```python
from build123d import *

# Parameters (mm, degrees)
BOSS_EXTRUDE1_DEPTH    = 152.4
CONVERT_SOLID1_START   = -152.4
CONVERT_SOLID1_DEPTH   = 152.4
CONVERT_SOLID1_2_DEPTH = 152.4
SKETCH6_W              = 60.654765258
SKETCH6_H              = 35.589797731
CUT_EXTRUDE1_DEPTH     = 230.810351377
SKETCH7_W              = 82.570052287
SKETCH7_H              = 50.8
CUT_EXTRUDE2_DEPTH     = 180.914674499


# Read off the part's stored shape, not the designer's step: Convert-Solid1
with BuildPart() as part:
    # Sketch1 → Boss-Extrude1 (new body)
    with BuildSketch(Plane.XY):
        Polygon((-82.55, 0), (-82.55, 48.26), (82.55, 48.26), (82.55, 0), (81.28, 0), (81.28, 46.99), (-81.28, 46.99), (-81.28, 0), align=None)
    extrude(amount=-BOSS_EXTRUDE1_DEPTH)

    # Convert-Solid1 outline → Convert-Solid1 (cut)
    with BuildSketch(Plane.XY.offset(CONVERT_SOLID1_START)):
        with BuildLine():
            Line((82.55, 48.26), (80.01, 48.26))
            ThreePointArc((80.01, 48.26), (81.806051224, 47.516051224), (82.55, 45.72))
            Line((82.55, 45.72), (82.55, 48.26))
        make_face()
        with BuildLine():
            ThreePointArc((-82.55, 45.72), (-81.806051224, 47.516051224), (-80.01, 48.26))
            Line((-80.01, 48.26), (-82.55, 48.26))
            Line((-82.55, 48.26), (-82.55, 45.72))
        make_face()
    extrude(amount=CONVERT_SOLID1_DEPTH, mode=Mode.SUBTRACT)

    # Convert-Solid1 2 outline → Convert-Solid1 2 (add)
    with BuildSketch(Plane.XY.offset(CONVERT_SOLID1_START)):
        with BuildLine():
            Line((81.28, 46.99), (80.01, 46.99))
            ThreePointArc((80.01, 46.99), (80.908025612, 46.618025612), (81.28, 45.72))
            Line((81.28, 45.72), (81.28, 46.99))
        make_face()
        with BuildLine():
            ThreePointArc((-81.28, 45.72), (-80.908025612, 46.618025612), (-80.01, 46.99))
            Line((-80.01, 46.99), (-81.28, 46.99))
            Line((-81.28, 46.99), (-81.28, 45.72))
        make_face()
    extrude(amount=CONVERT_SOLID1_2_DEPTH)

    # Sketch6 → Cut-Extrude1 (cut, through all)
    with BuildSketch(Plane.ZY.offset(82.55)):
        with Locations((-1.422617371, 1.255101135)):
            Rectangle(SKETCH6_W, SKETCH6_H)
    extrude(amount=-CUT_EXTRUDE1_DEPTH, mode=Mode.SUBTRACT)

    # Sketch7 → Cut-Extrude2 (cut, through all)
    with BuildSketch(Plane(origin=(0, 48.26, 0), x_dir=(1, 0, 0), z_dir=(0, 1, 0))):
        with Locations((73.035026144, 91.44)):
            Rectangle(SKETCH7_W, SKETCH7_H)
    extrude(amount=-CUT_EXTRUDE2_DEPTH, mode=Mode.SUBTRACT)


solid = part.part
```
Can you work these out from the model? Positions are in its coordinate system, mm. A direction names the side the tool comes from. Coordinates: 2 decimals unless noted, no trailing zeros. Loops run counter-clockwise (first coordinate to the right, second up) from the corner with the lowest first, then second, coordinate; pieces in that order, holes last. Notation, with made-up numbers: (-6, 73.5) - (12, 73.5) arc R20 ccw to (12, 112.5) - close; hole circle Ø9 at (42.25, 29.5). An arc over 180 degrees is marked (long way). Answer as CSV lines item,"result". Start each with the question number.
1) I need wall thicknesses on line 1 (X direction, y = 22, z = -141.5); line 2 (Y direction, x = 25.5, z = -81); line 3 (X direction, y = 40, z = -95). Which ranges of each line are inside material? Lowest first, please. Write a range as from..to.
2) Which directions (+Z, -Z, +X, -X, +Y, -Y) give clear straight access to the entire face, cutting with the end or side of a thin tool? Please do faces 4 (the flat face through (68.3, 47.5, -66.04)), 5 (the flat face through (1, 46.99, -75)), 6 (the flat face through (82.55, 28, -40)).
3) Suppose I cut it at C-C (y = 35.5). Please give me the cut outline in (x, z).
4) Suppose I cut it at A-A (y = 8). Please give me the cut outline in (x, z).
5) Thinking about a two-plate mould opening in X: for faces 1 (the flat face through (81.28, 23, -134)), 2 (the flat face through (68.3, 47.5, -116.84)), 3 (the flat face through (-82.55, 23, -75)), which applies, pulls with the +X half, pulls with the -X half, needs draft (parallel to the pull), parting line crosses it, or undercut?
6) For pin 1 (1 mm diameter, centred on x = 4.5, z = -50, fed in from -Y); pin 2 (1 mm diameter, centred on x = -82, z = -11, fed in from -Y); pin 3 (1.4 mm diameter, centred on x = -82, y = 7, fed in from +Z), each with a flat end and sliding along its axis, tell me the tip position at first contact or that it passes through.
7) Suppose I cut it at D-D (x = -68). Please give me the cut outline in (y, z), plus the area to 3 significant figures.
8) Suppose I cut it at B-B (z = -56.5). Please give me the cut outline in (x, y), plus the area to 3 significant figures.
Check result:
1,line 1,"x = -82.55..-81.28, 81.28..82.55"
1,line 2,"y = 46.99..48.26"
1,line 3,"x = -82.55..-81.28"
2,face 4,"+X, +Y, -Y"
2,face 5,"+Z, -Z, -Y"
2,face 6,"+Z, -Z, +X, +Y, -Y"
3,outline,"(-82.55, -152.4) - (-81.28, -152.4) - (-81.28, 0) - (-82.55, 0) - close; (81.28, -152.4) - (82.55, -152.4) - (82.55, -116.84) - (81.28, -116.84) - close; (81.28, -66.04) - (82.55, -66.04) - (82.55, 0) - (81.28, 0) - close"
4,outline,"(-82.55, -152.4) - (-81.28, -152.4) - (-81.28, -31.75) - (-82.55, -31.75) - close; (81.28, -152.4) - (82.55, -152.4) - (82.55, -116.84) - (81.28, -116.84) - close; (81.28, -66.04) - (82.55, -66.04) - (82.55, -31.75) - (81.28, -31.75) - close"
5,face 1,"undercut"
5,face 2,"needs draft"
5,face 3,"pulls with the -X half"
6,pin 1,"stops at y = 46.99"
6,pin 2,"stops at y = 19.05"
6,pin 3,"stops at z = -31.75"
7,outline,"(46.99, -152.4) - (48.26, -152.4) - (48.26, 0) - (46.99, 0) - close"
7,area,"194 mm²"
8,outline,"(-82.55, 0) - (-81.28, 0) - (-81.28, 45.72) arc R1.27 cw to (-80.01, 46.99) - (80.01, 46.99) arc R1.27 cw to (81.28, 45.72) - (81.28, 0) - (82.55, 0) - (82.55, 45.72) arc R2.54 ccw to (80.01, 48.26) - (-80.01, 48.26) arc R2.54 ccw to (-82.55, 45.72) - close"
8,area,"327 mm²"
